Read the model definition and answer for the solid it produces. Units are mm, in the model's axes. A direction names the side the tool comes from. Round coordinates to 2 decimals unless told otherwise and drop trailing zeros. Loops run counter-clockwise (first coordinate to the right, second up) from the corner with the lowest first, then second, coordinate; pieces in that order, holes last. Notation, with made-up numbers: (43.25, 82.5) -> (77.25, 82.5) arc R20 cw to (77.25, 108.5) -> close; hole circle Ø6 at (76, 35.5). An arc over 180 degrees is marked (long way). Put each result on its own line as item: value.
from build123d import *

# Parameters (mm, degrees)
SKETCH1_R           = 0.75
BOSS_EXTRUDE1_DEPTH = 18
SKETCH2_R           = 0.5
BOSS_EXTRUDE2_DEPTH = 0.4
SKETCH3_R           = 0.5
BOSS_EXTRUDE3_DEPTH = 0.4


with BuildPart() as part:
    # Sketch1 → Boss-Extrude1 (new body)
    with BuildSketch(Plane(origin=(0, 0, 0), x_dir=(0, 0, -1), z_dir=(1, 0, 0))):
        Circle(SKETCH1_R)
    extrude(amount=BOSS_EXTRUDE1_DEPTH)

    # Sketch2 → Boss-Extrude2 (add)
    with BuildSketch(Plane(origin=(18, 0, 0), x_dir=(0, 0, -1), z_dir=(1, 0, 0))):
        Circle(SKETCH2_R)
    extrude(amount=BOSS_EXTRUDE2_DEPTH)

    # Sketch3 → Boss-Extrude3 (add)
    with BuildSketch(Plane.ZY):
        Circle(SKETCH3_R)
    extrude(amount=BOSS_EXTRUDE3_DEPTH)


solid = part.part
Item 1: Which of the six approach directions +Z, -Z, +X, -X, +Y, -Y give full straight-line access (tool end or side, diameter ignored) to faces 1 (the cylindrical face through (-0.197, -0.488, -0.108)), 2 (the cylindrical face through (18.197, -0.488, 0.108)), 3 (the cylindrical face through (8.87, 0.03, 0.75))?
Derived:
face 1: -X
face 2: +X
face 3: +X, -X
Item 2: Find the intervals of material crossed by line 1 along X through (y, z) = (0.6, -0.35); line 2 along Z through (x, y) = (17, -0.05); line 3 along Y through (x, z) = (6.5, 0.15), in increasing order.
Derived:
line 1: x = 0 to 18
line 2: z = -0.75 to 0.75
line 3: y = -0.73 to 0.73
Item 3: The part is cut by section B-B (x = 5.5). Determine the outline of the cut face in (y, z), then the cut area to 3 significant figures.
Derived:
outline: circle Ø1.5 at (0, 0)
area: 1.77 mm^2
Item 4: The part is cut by section A-A (z = -0.1). Determine the outline of the cut face in (x, y), then the cut area to 3 significant figures.
Derived:
outline: (-0.4, -0.49) -> (0, -0.49) -> (0, -0.74) -> (18, -0.74) -> (18, -0.49) -> (18.4, -0.49) -> (18.4, 0.49) -> (18, 0.49) -> (18, 0.74) -> (0, 0.74) -> (0, 0.49) -> (-0.4, 0.49) -> close
area: 27.5 mm^2
